For this review, use the dimensioned drawing (mm, ordinates from the lowest corner) and the shaded views. Round coordinates to 2 decimals unless told otherwise and drop trailing zeros. Order: outer loops, then holes, each group sorted by start corner. A loop starts at its lowest first (then second) coordinate and runs counter-clockwise, first axis right, second up. Notation, with made-up numbers: (64.25, -25) - (123.25, -25) arc R18 ccw to (123.25, 1) - close; hole circle Ø1 at (43.25, 28). An arc over 180 degrees is marked (long way). Write each question's results on one line, items separated by ' | '. Start each with the question number.
(1) Draft analysis for pull direction X (two halves, no side actions). For the marked faces 1, 2 and 3, state which applies: pulls with the +X half, pulls with the -X half, needs draft (parallel to the pull), parting line crosses it, or undercut.
(2) Take a section at C-C, the plane x = 6. Give the boundary of the cut face in (y, z).
(3) Take a section at D-D, the plane z = 55. Give the boundary of the cut face in (x, y).
(4) Take a section at A-A, the plane x = 30. Give the boundary of the cut face in (y, z), plus the area to 3 significant figures.
(5) For L1, parallel to X at y = 16, z = 30; L2, parallel to X at y = 5, z = 30, list the stretches that pass through material, from the lowest coordinate up. Write a range as from..to.
(6) Take a section at B-B, the plane z = 30. Give the boundary of the cut face in (x, y).
(7) Insertion check: pin 1 Ø1.5 at (x, y) = (22, 3.5) entering from +Z; pin 2 Ø3 at (y, z) = (10, 47) entering from -X; pin 3 Ø12 at (y, z) = (22.5, 11.5) entering from -X. Each pin has a flat end and moves straight along its axis. Give the tip position at first contact, or say it passes through.
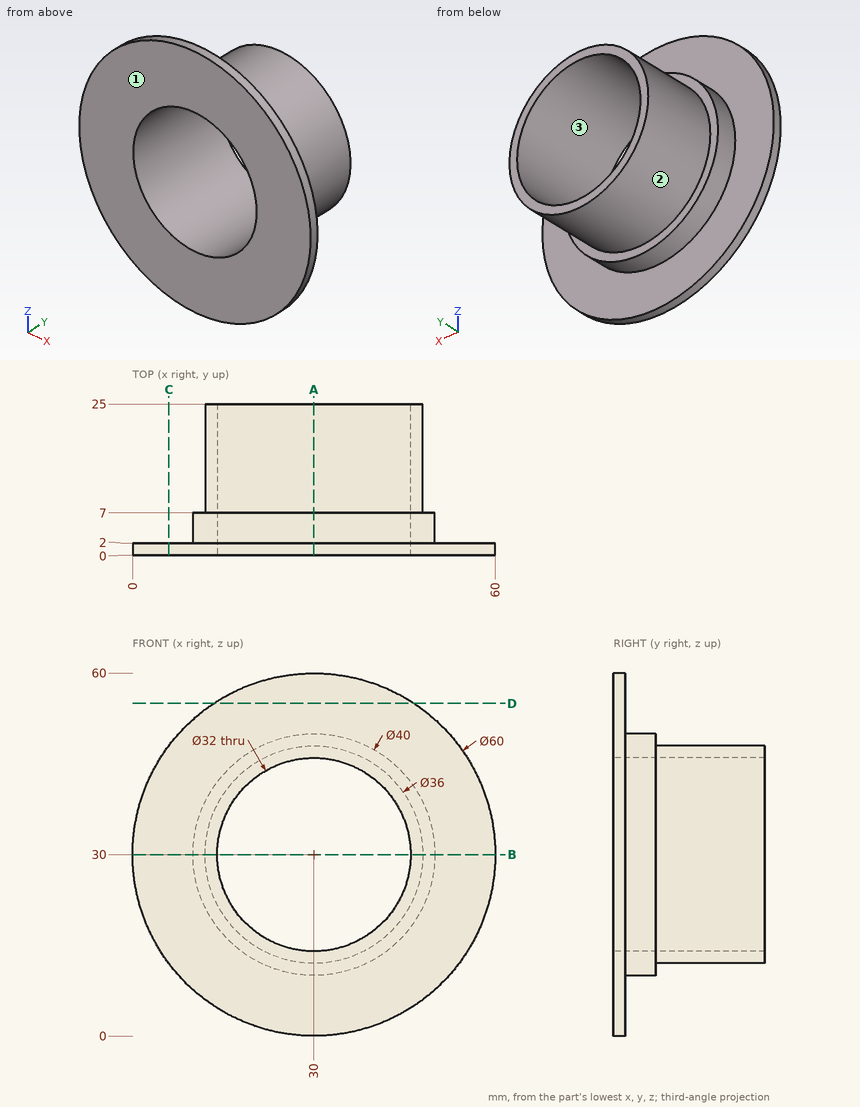
Results below:
1) face 1: needs draft | face 2: parting line crosses it | face 3: undercut
2) outline: (0, 12) - (2, 12) - (2, 48) - (0, 48) - close
3) outline: (13.42, 0) - (46.58, 0) - (46.58, 2) - (13.42, 2) - close
4) outline: (0, 0) - (2, 0) - (2, 10) - (7, 10) - (7, 12) - (25, 12) - (25, 14) - (0, 14) - close; (0, 46) - (25, 46) - (25, 48) - (7, 48) - (7, 50) - (2, 50) - (2, 60) - (0, 60) - close | area: 168 mm^2
5) L1: x = 12..14, 46..48 | L2: x = 10..14, 46..50
6) outline: (0, 0) - (14, 0) - (14, 25) - (12, 25) - (12, 7) - (10, 7) - (10, 2) - (0, 2) - close; (46, 0) - (60, 0) - (60, 2) - (50, 2) - (50, 7) - (48, 7) - (48, 25) - (46, 25) - close
7) pin 1: stops at z = 48.64 | pin 2: stops at x = 20.85 | pin 3: stops at x = 17.05
